from build123d import *

# Parameters (mm, degrees)
CROQUIS1_R                 = 6.5
SALIENTE_EXTRUIR1_DEPTH    = 45
CROQUIS2_R                 = 5
CORTAR_EXTRUIR1_DEPTH      = 15
CORTAR_EXTRUIR2_REACH      = 47.929
CROQUIS4_R                 = 6.5
SALIENTE_EXTRUIR2_DEPTH    = 15
CORTAR_EXTRUIR3_REACH      = 62.7
CROQUIS5_R                 = 2.5
CORTAR_EXTRUIR4_DEPTH      = 61.700082372
CORTAR_EXTRUIR4_DEPTH_BACK = 61.700082372
CROQUIS7_R                 = 1.5
CORTAR_EXTRUIR5_DEPTH      = 61.700082493
CORTAR_EXTRUIR5_DEPTH_BACK = 61.700082493
CROQUIS8_R                 = 1.5


with BuildPart() as part:
    # Croquis1 → Saliente-Extruir1 (new body)
    with BuildSketch(Plane.XY):
        with Locations(Location((0, 0, 0), (0, 0, 180))):
            Circle(CROQUIS1_R)
    extrude(amount=SALIENTE_EXTRUIR1_DEPTH)

    # Croquis2 → Cortar-Extruir1 (cut)
    with BuildSketch(Plane(origin=(0, 0, 0), x_dir=(-1, 0, 0), z_dir=(0, 0, -1))):
        Circle(CROQUIS2_R)
    extrude(amount=-CORTAR_EXTRUIR1_DEPTH, mode=Mode.SUBTRACT)

    # Croquis3 → Cortar-Extruir2 (cut, up to next)
    with BuildSketch(Plane.XY.offset(45), mode=Mode.PRIVATE) as cortar_extruir2_sk1:
        Polygon((-5, 0), (-2.5, -4.330127019), (2.5, -4.330127019), (5, 0), (2.5, 4.330127019), (-2.5, 4.330127019), align=None)
    cortar_extruir2_tool1 = extrude(cortar_extruir2_sk1.sketch, amount=-CORTAR_EXTRUIR2_REACH, mode=Mode.PRIVATE) & part.part
    add(cortar_extruir2_tool1.solids().sort_by_distance((0, 0, 45))[0], mode=Mode.SUBTRACT)

    # Croquis4 → Saliente-Extruir2 (add)
    with BuildSketch(Plane.XY.offset(45)):
        with Locations(Location((0, 0, 0), (0, 0, 180))):
            Circle(CROQUIS4_R)
    extrude(amount=SALIENTE_EXTRUIR2_DEPTH)

    # Croquis5 → Cortar-Extruir3 (cut, up to next)
    with BuildSketch(Plane.XY.offset(60), mode=Mode.PRIVATE) as cortar_extruir3_sk1:
        Circle(CROQUIS5_R)
    cortar_extruir3_tool1 = extrude(cortar_extruir3_sk1.sketch, amount=-CORTAR_EXTRUIR3_REACH, mode=Mode.PRIVATE) & part.part
    add(cortar_extruir3_tool1.solids().sort_by_distance((0, 0, 60))[0], mode=Mode.SUBTRACT)

    # Croquis7 → Cortar-Extruir4 (cut, two sides: drawn at the far end of the back side and taken through both)
    with BuildSketch(Plane(origin=(0, 0, 0), x_dir=(0, 0, -1), z_dir=(1, 0, 0)).offset(-CORTAR_EXTRUIR4_DEPTH_BACK)):
        with Locations((-53, 0)):
            Circle(CROQUIS7_R)
    extrude(amount=CORTAR_EXTRUIR4_DEPTH + CORTAR_EXTRUIR4_DEPTH_BACK, mode=Mode.SUBTRACT)

    # Croquis8 → Cortar-Extruir5 (cut, two sides: drawn at the far end of the back side and taken through both)
    with BuildSketch(Plane(origin=(0, 0, 0), x_dir=(1, 0, 0), z_dir=(0, 1, 0)).offset(-CORTAR_EXTRUIR5_DEPTH_BACK)):
        with Locations(Location((0, -30, 0), (0, 0, 270))):
            Circle(CROQUIS8_R)
    extrude(amount=CORTAR_EXTRUIR5_DEPTH + CORTAR_EXTRUIR5_DEPTH_BACK, mode=Mode.SUBTRACT)


solid = part.part
Design review of the part built by this model. Coordinates are the model's own, in mm. A direction names the side the tool comes from. Round coordinates to 2 decimals unless told otherwise and drop trailing zeros. Loops run counter-clockwise (first coordinate to the right, second up) from the corner with the lowest first, then second, coordinate; pieces in that order, holes last. Notation, with made-up numbers: (10.25, 20) - (31.25, 20) arc R29 ccw to (31.25, 44) - close; hole circle Ø3 at (22, -37.75). An arc over 180 degrees is marked (long way). One line per question, with ' | ' between items.
1. We need section D-D, the plane x = -3.25. State the section outline as (y, z) points.
Results are:
outline: (-5.63, 0) - (-3.8, 0) - (-3.8, 15) - (-3.03, 15) - (-3.03, 45) - (3.03, 45) - (3.03, 15) - (3.8, 15) - (3.8, 0) - (5.63, 0) - (5.63, 60) - (-5.63, 60) - close; hole circle Ø3 at (0, 53)
2. Clearance check with flat-ended pins moving along their axes: P1, Ø2, axis at x = 3, z = 33, coming from the +Y side; P2, Ø2.5, axis at x = 1.5, y = 0, coming from the -Z side; P3, Ø0.7, axis at x = -0.5, y = -4.5, coming from the -Z side. State where each tip first meets the part, or that it passes through.
Results are:
P1: stops at y = 6.18 | P2: stops at z = 45 | P3: stops at z = 15
3. We need section B-B, the plane z = 26.5. State the section outline as (x, y) points, and give its area (3 significant figures).
Results are:
outline: circle Ø13 at (0, 0); hole (-5, 0) - (-2.5, -4.33) - (2.5, -4.33) - (5, 0) - (2.5, 4.33) - (-2.5, 4.33) - close | area: 67.8 mm²
4. For faces 5 (the face through (-4.282, -0.575, 51.614)), 6 (the face through (4, -2.3, 15)), list the 3-axis set-ups (+Z, -Z, +X, -X, +Y, -Y) from which the entire face can be reached by the end or side of a thin tool; tool diameter is ignored.
Results are:
face 5: +X, -X | face 6: -Z
5. We need section A-A, the plane x = 0. State the section outline as (y, z) points, and give its area (3 significant figures).
Results are:
outline: (-6.5, 0) - (-5, 0) - (-5, 15) - (-4.33, 15) - (-4.33, 28.5) - (-6.5, 28.5) - close; (-6.5, 31.5) - (-4.33, 31.5) - (-4.33, 45) - (-2.5, 45) - (-2.5, 60) - (-6.5, 60) - close; (2.5, 45) - (4.33, 45) - (4.33, 31.5) - (6.5, 31.5) - (6.5, 60) - (2.5, 60) - close; (4.33, 15) - (5, 15) - (5, 0) - (6.5, 0) - (6.5, 28.5) - (4.33, 28.5) - close | area: 282 mm²
6. For L1, parallel to Z at x = 0, y = 4.8; L2, parallel to Z at x = -4, y = 2.5; L3, parallel to X at y = -6, z = 53, list the stretches that pass through material, from the lowest coordinate up. Write a range as [from, to].
Results are:
L1: z = [15, 28.5], [31.5, 60] | L2: z = [15, 60] | L3: x = [-2.5, 2.5]
7. We need section C-C, the plane z = 53. State the section outline as (x, y) points, and give its area (3 significant figures).
Results are:
outline: (-6.32, -1.5) arc R6.5 ccw to (6.32, -1.5) - (2, -1.5) arc R2.5 cw to (-2, -1.5) - close; (-6.32, 1.5) - (-2, 1.5) arc R2.5 cw to (2, 1.5) - (6.32, 1.5) arc R6.5 ccw to start | area: 88.5 mm²
8. Draft analysis for pull direction Z (two halves, no side actions). For faces 1 (the face through (1.487, 5.402, 29.805)), 2 (the face through (-3, 0, 60)), 3 (the face through (-3.77, -2.13, 30.21)), 4 (the face through (-4, -2.3, 15)), state which applies: released by +Z, released by -Z, zero draft, split by the parting line, or undercut.
Results are:
face 1: undercut | face 2: released by +Z | face 3: zero draft | face 4: released by -Z
